Part model, mm, in its own coordinate system. A direction names the side the tool comes from. Coordinates: 2 decimals unless noted, no trailing zeros. Loops run counter-clockwise (first coordinate to the right, second up) from the corner with the lowest first, then second, coordinate; pieces in that order, holes last. Notation, with made-up numbers: M 65,56 L 108,56 A12 cw 108,67 Z; hole C -28,59.25 d11. An arc over 180 degrees is marked long. Use a Markdown table: item, result. Add a question column.
1) Pin check, flat tips, straight feed: pin 1 Ø1 at (y, z) = (1, -16.5) entering from +X (3 decimals); pin 2 Ø1 at (x, y) = (13.5, 1) entering from +Z. Stop position of each tip, or through.
2) Tool access for faces 4 (the cylindrical face through (15.246, 0.805, -20.911)), 5 (the flat face through (16, 0, -21)): list every direction of +Z, -Z, +X, -X, +Y, -Y with a clear straight run to the whole face (end or side of a thin tool).
3) Band-saw the part on A-A (y = 1.3). State how many separate pieces and enclosed holes the cut face has, plus the area to 3 significant figures.
4) Wall check: probe 1 along Z at (x, y) = (15.75, 0.8); probe 2 along Z at (x, y) = (13.25, 1.4); probe 3 along X at (y, z) = (0.3, -21.25). Give the ranges that are in metal, low to high. Write a range as from..to.
5) Pull direction X, two halves, no side cores. Call faces 1 (the flat face through (12, 3, -15.61)), 2 (the cylindrical face through (13.424, 0.805, -16.625)), 3 (the flat face through (17.71, 3, -21)): released by +X, released by -X, zero draft, split by the parting line, or undercut.
6) Band-saw the part on D-D (z = -23.25). List the corners of the cut face in (x, y), plus the area to 3 significant figures.
from build123d import *

# Parameters (mm, degrees)
SKETCH3_W           = 10.7
SKETCH3_H           = 10.7
BOSS_EXTRUDE2_DEPTH = 2.41
SKETCH5_R           = 1.115
BOSS_EXTRUDE3_DEPTH = 1.5875


with BuildPart() as part:
    # Sketch3 → Boss-Extrude2 (new body)
    with BuildSketch(Plane(origin=(0, 1.5875, 0), x_dir=(-1, 0, 0), z_dir=(0, 1, 0))):
        with Locations((-12.36, -20.96)):
            Rectangle(SKETCH3_W, SKETCH3_H)
    extrude(amount=BOSS_EXTRUDE2_DEPTH)

    # Sketch5 → Boss-Extrude3 (add)
    with BuildSketch(Plane.XZ.offset(-1.5875)):
        with Locations((16.36, -24.96)):
            Circle(SKETCH5_R)
        with Locations((12.36, -24.96)):
            Circle(SKETCH5_R)
        with Locations((8.36, -24.96)):
            Circle(SKETCH5_R)
        with Locations((16.36, -20.96)):
            Circle(SKETCH5_R)
        with Locations((12.36, -20.96)):
            Circle(SKETCH5_R)
        with Locations((8.36, -20.96)):
            Circle(SKETCH5_R)
        with Locations((16.36, -16.96)):
            Circle(SKETCH5_R)
        with Locations((12.36, -16.96)):
            Circle(SKETCH5_R)
        with Locations((8.36, -16.96)):
            Circle(SKETCH5_R)
    extrude(amount=BOSS_EXTRUDE3_DEPTH)


solid = part.part
Entries:
| question | item | result |
|---|---|---|
| 1 | pin 1 | x = 17.475 |
| 1 | pin 2 | z = -16.05 |
| 2 | face 4 | -Y |
| 2 | face 5 | +Z, -Z, +X, -X, -Y |
| 3 | separate pieces | 9 |
| 3 | enclosed holes | 0 |
| 3 | area | 35.2 mm2 |
| 4 | probe 1 | -25.89..-24.03, -21.89..-20.03, -17.89..-16.03 |
| 4 | probe 2 | -25.63..-24.29, -21.63..-20.29, -17.63..-16.29 |
| 4 | probe 3 | 7.28..9.44, 11.28..13.44, 15.28..17.44 |
| 5 | face 1 | zero draft |
| 5 | face 2 | undercut |
| 5 | face 3 | released by +X |
| 6 | outline | M 7.01,1.59 L 17.71,1.59 L 17.71,4 L 7.01,4 Z |
| 6 | area | 25.8 mm2 |
